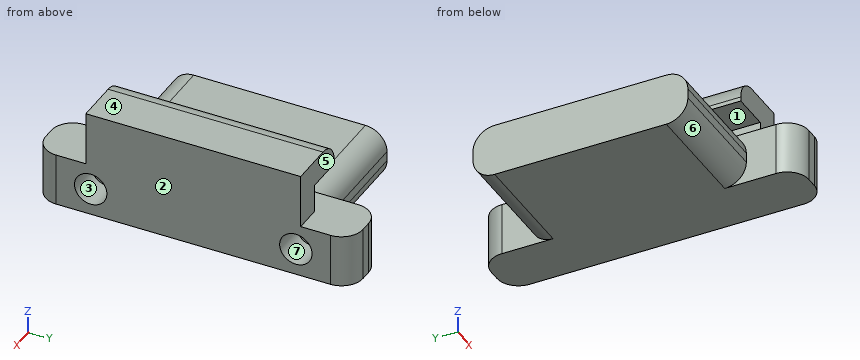
from build123d import *

# Parameters (mm, degrees)
EXTRUDE_1_DEPTH     = 4.9
FILLET_1_R          = 2
SKETCH_3_R          = 1.5
CUT_EXTRUDE_1_DEPTH = 3
SKETCH_4_W          = 5
SKETCH_4_H          = 19.9
EXTRUDE_2_DEPTH     = 5
SKETCH_5_W          = 2.5
SKETCH_5_H          = 2.6
CUT_EXTRUDE_2_DEPTH = 31.755202812
FILLET_3_R          = 2
SKETCH_6_W          = 2.4
SKETCH_6_H          = 19.9
EXTRUDE_3_DEPTH     = 1
FILLET_4_R          = 2


with BuildPart() as part:
    # 草图2 → 凸台-拉伸1 (new body)
    with BuildSketch(Plane.XY):
        Polygon((0, 0), (0, 19.9), (10.5, 19.9), (10.5, 24.65), (15.5, 24.65), (15.5, -4.75), (10.5, -4.75), (10.5, 0), align=None)
    extrude(amount=EXTRUDE_1_DEPTH)

    # 圆角1
    fillet_1_edges = [part.edges().sort_by_distance(p)[0] for p in [
        (5.25, 0, 0),
        (5.25, 19.9, 4.9),
        (5.25, 0, 4.9),
        (5.25, 19.9, 0),
    ]]
    fillet(fillet_1_edges, radius=FILLET_1_R)

    # 草图3 → 切除-拉伸1 (cut)
    with BuildSketch(Plane(origin=(15.5, 0, 0), x_dir=(0, 0, -1), z_dir=(1, 0, 0))):
        with Locations(Location((-2.5, 19.45, 0), (0, 0, 90))):
            Circle(SKETCH_3_R)
        with Locations(Location((-2.5, 0.45, 0), (0, 0, 270))):
            Circle(SKETCH_3_R)
    extrude(amount=-CUT_EXTRUDE_1_DEPTH, mode=Mode.SUBTRACT)

    # 草图4 → 凸台-拉伸2 (add)
    with BuildSketch(Plane.XY.offset(4.9)):
        with Locations((13, 9.95)):
            Rectangle(SKETCH_4_W, SKETCH_4_H)
    extrude(amount=EXTRUDE_2_DEPTH)

    # 草图5 → 切除-拉伸2 (cut, through all)
    with BuildSketch(Plane(origin=(0, 19.9, 0), x_dir=(1, 0, 0), z_dir=(0, 1, 0))):
        with Locations((11.75, -6.2)):
            Rectangle(SKETCH_5_W, SKETCH_5_H)
    extrude(amount=-CUT_EXTRUDE_2_DEPTH, mode=Mode.SUBTRACT)

    # 圆角3
    fillet_3_edges = [part.edges().sort_by_distance(p)[0] for p in [
        (10.5, 24.65, 2.45),
        (15.5, 24.65, 2.45),
        (15.5, -4.75, 2.45),
        (10.5, -4.75, 2.45),
    ]]
    fillet(fillet_3_edges, radius=FILLET_3_R)

    # 草图6 → 凸台-拉伸3 (add)
    with BuildSketch(Plane.ZY.offset(-10.5)):
        with Locations((8.7, 9.95)):
            Rectangle(SKETCH_6_W, SKETCH_6_H)
    extrude(amount=EXTRUDE_3_DEPTH)

    # 圆角4
    fillet_4_edges = [part.edges().sort_by_distance(p)[0] for p in [
        (9.5, 9.95, 9.9),
    ]]
    fillet(fillet_4_edges, radius=FILLET_4_R)


solid = part.part
Input: part model. Units: mm. Frame: model coordinates. Face numbers are marked on the shaded views. A direction names the side the tool comes from. Coordinates: 2 decimals unless noted, no trailing zeros. Loops run counter-clockwise (first coordinate to the right, second up) from the corner with the lowest first, then second, coordinate; pieces in that order, holes last. Notation, with made-up numbers: (78, -23) -> (110, -23) arc R18 ccw to (110, -3) -> close; hole circle Ø3 at (24, -36.5). An arc over 180 degrees is marked (long way). One line per item, written item: value.
(1) Cut plane A-A (x = 8.5). Output: boundary loops of the cut face in (y, z), then the cut area to 3 significant figures.
Answer below:
outline: (0, 2) arc R2 ccw to (2, 0) -> (17.9, 0) arc R2 ccw to (19.9, 2) -> (19.9, 2.9) arc R2 ccw to (17.9, 4.9) -> (2, 4.9) arc R2 ccw to (0, 2.9) -> close
area: 94.1 mm2
(2) Pin query (flat end, axial travel): pin 1 Ø0.5 at (x, z) = (5, 2.5) entering from +Y; pin 2 Ø2 at (x, z) = (10, 4.5) entering from +Y; pin 3 Ø0.9 at (y, z) = (20, 3) entering from +X. Return the tip coordinate at first contact, or that it passes through.
Answer below:
pin 1: stops at y = 19.9
pin 2: stops at y = 23.97
pin 3: stops at x = 12.5
(3) Set-up query: the marked faces 1, 2 and 3. Return all of +Z, -Z, +X, -X, +Y, -Y with unobstructed straight access to the full face (end or side cutting, diameter ignored); none if empty.
Answer below:
face 1: -X, +Y, -Y
face 2: +Z, -Z, +X, +Y, -Y
face 3: +X
(4) Cut plane C-C (y = 6.25). Output: boundary loops of the cut face in (x, z).
Answer below:
outline: (0, 0) -> (15.5, 0) -> (15.5, 9.9) -> (11.5, 9.9) arc R2 ccw to (9.5, 7.9) -> (9.5, 7.5) -> (13, 7.5) -> (13, 4.9) -> (0, 4.9) -> close
(5) Ray query, line 1 along Z through (x, y) = (14.85, 0.45); line 2 along Z through (x, y) = (12.5, 9.75); line 3 along Y through (x, z) = (14.75, 1.5). Return the intervals inside material, ascending.
Answer below:
line 1: z = 0 to 1, 4 to 9.9
line 2: z = 0 to 4.9, 7.5 to 9.9
line 3: y = -4.31 to -0.67, 1.57 to 18.33, 20.57 to 24.21
(6) Cut plane B-B (z = 2.5). Output: boundary loops of the cut face in (x, y), then the cut area to 3 significant figures.
Answer below:
outline: (0, 0) -> (10.5, 0) -> (10.5, -2.75) arc R2 ccw to (12.5, -4.75) -> (13.5, -4.75) arc R2 ccw to (15.5, -2.75) -> (15.5, -1.05) -> (12.5, -1.05) -> (12.5, 1.95) -> (15.5, 1.95) -> (15.5, 17.95) -> (12.5, 17.95) -> (12.5, 20.95) -> (15.5, 20.95) -> (15.5, 22.65) arc R2 ccw to (13.5, 24.65) -> (12.5, 24.65) arc R2 ccw to (10.5, 22.65) -> (10.5, 19.9) -> (0, 19.9) -> close
area: 335 mm2
(7) Draft query along Z for the marked faces 4, 5, 6 and 7. Return one class per face: pulls with the +Z half, pulls with the -Z half, needs draft (parallel to the pull), parting line crosses it, or undercut.
Answer below:
face 4: pulls with the +Z half
face 5: needs draft
face 6: pulls with the -Z half
face 7: undercut
(8) Cut plane D-D (z = 4.5). Output: boundary loops of the cut face in (x, y).
Answer below:
outline: (0, 0.8) -> (10.5, 0.8) -> (10.5, -2.75) arc R2 ccw to (12.5, -4.75) -> (13.5, -4.75) arc R2 ccw to (15.5, -2.75) -> (15.5, 22.65) arc R2 ccw to (13.5, 24.65) -> (12.5, 24.65) arc R2 ccw to (10.5, 22.65) -> (10.5, 19.1) -> (0, 19.1) -> close
